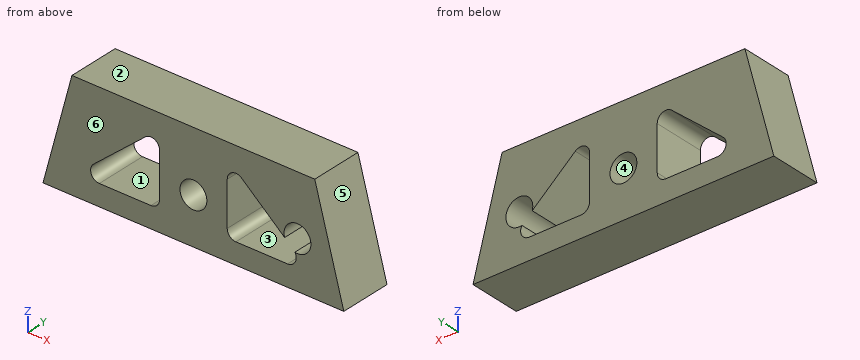
```python
from build123d import *

# Parameters (mm, degrees)
EXTRUDE_1_DEPTH     = 1
EXTRUDE_START       = 5
EXTRUDE_2_DEPTH     = 5
CUT_EXTRUDE_1_REACH = 25.286
SKETCH_2_R          = 1.55
SKETCH_3_R          = 1.55
CUT_EXTRUDE_2_DEPTH = 6


with BuildPart() as part:
    # 草图1 → 凸台-拉伸1 (new body)
    with BuildSketch(Plane(origin=(0, 0, 0), x_dir=(1, 0, 0), z_dir=(0, 1, 0))):
        Polygon((-0.862647581, -12.802774991), (12.834963402, -12.802774991), (16.186049163, -0.402774991), (-18.501877746, -0.402774991), (-15.165036598, -12.802774991), align=None)
        with BuildLine():
            Line((-5.055880083, -8.924536815), (-5.055880083, -3.827423548))
            ThreePointArc((-5.055880083, -3.827423548), (-5.348773301, -3.120316767), (-6.055880083, -2.827423548))
            Line((-6.055880083, -2.827423548), (-12.010923306, -2.827423548))
            ThreePointArc((-12.010923306, -2.827423548), (-12.948929404, -3.480804795), (-12.661184313, -4.587134428))
            Line((-12.661184313, -4.587134428), (-6.70614109, -9.684247695))
            ThreePointArc((-6.70614109, -9.684247695), (-5.63770608, -9.832903758), (-5.055880083, -8.924536815))
        make_face(mode=Mode.SUBTRACT)
        with BuildLine():
            Line((10.34535573, -4.587134428), (4.390312507, -9.684247695))
            ThreePointArc((4.390312507, -9.684247695), (3.321877497, -9.832903758), (2.740051499, -8.924536815))
            Line((2.740051499, -8.924536815), (2.740051499, -3.827423548))
            ThreePointArc((2.740051499, -3.827423548), (3.032944718, -3.120316767), (3.740051499, -2.827423548))
            Line((3.740051499, -2.827423548), (9.695094722, -2.827423548))
            ThreePointArc((9.695094722, -2.827423548), (10.63310082, -3.480804795), (10.34535573, -4.587134428))
        make_face(mode=Mode.SUBTRACT)
    extrude(amount=-EXTRUDE_1_DEPTH)

    # 草图1<8> → 凸台-拉伸2 (add)
    with BuildSketch(Plane(origin=(0, 0, 0), x_dir=(1, 0, 0), z_dir=(0, 1, 0)).offset(EXTRUDE_START)):
        Polygon((-0.862647581, -12.802774991), (12.834963402, -12.802774991), (16.186049163, -0.402774991), (-18.501877746, -0.402774991), (-15.165036598, -12.802774991), align=None)
        with BuildLine():
            Line((-5.055880083, -8.924536815), (-5.055880083, -3.827423548))
            ThreePointArc((-5.055880083, -3.827423548), (-5.348773301, -3.120316767), (-6.055880083, -2.827423548))
            Line((-6.055880083, -2.827423548), (-12.010923306, -2.827423548))
            ThreePointArc((-12.010923306, -2.827423548), (-12.948929404, -3.480804795), (-12.661184313, -4.587134428))
            Line((-12.661184313, -4.587134428), (-6.70614109, -9.684247695))
            ThreePointArc((-6.70614109, -9.684247695), (-5.63770608, -9.832903758), (-5.055880083, -8.924536815))
        make_face(mode=Mode.SUBTRACT)
        with BuildLine():
            Line((10.34535573, -4.587134428), (4.390312507, -9.684247695))
            ThreePointArc((4.390312507, -9.684247695), (3.321877497, -9.832903758), (2.740051499, -8.924536815))
            Line((2.740051499, -8.924536815), (2.740051499, -3.827423548))
            ThreePointArc((2.740051499, -3.827423548), (3.032944718, -3.120316767), (3.740051499, -2.827423548))
            Line((3.740051499, -2.827423548), (9.695094722, -2.827423548))
            ThreePointArc((9.695094722, -2.827423548), (10.63310082, -3.480804795), (10.34535573, -4.587134428))
        make_face(mode=Mode.SUBTRACT)
    extrude(amount=-EXTRUDE_2_DEPTH)

    # 草图2 → 切除-拉伸1 (cut, up to next)
    with BuildSketch(Plane(origin=(0, 5, 0), x_dir=(1, 0, 0), z_dir=(0, 1, 0)), mode=Mode.PRIVATE) as cut_extrude_1_sk1:
        with Locations(Location((-1.157914292, -5.802774991, 0), (0, 0, 270))):
            Circle(SKETCH_2_R)
    cut_extrude_1_tool1 = extrude(cut_extrude_1_sk1.sketch, amount=-CUT_EXTRUDE_1_REACH, mode=Mode.PRIVATE) & part.part
    add(cut_extrude_1_tool1.solids().sort_by_distance((-1.157914, 5, 5.802775))[0], mode=Mode.SUBTRACT)

    # 草图3 → 切除-拉伸2 (cut)
    with BuildSketch(Plane(origin=(0, 5, 0), x_dir=(1, 0, 0), z_dir=(0, 1, 0))):
        with Locations((10.842085708, -5.882306345)):
            Circle(SKETCH_3_R)
    extrude(amount=-CUT_EXTRUDE_2_DEPTH, mode=Mode.SUBTRACT)


solid = part.part
```
Model file for the job. Use its own axes, mm. Face numbers are marked on the shaded views. A direction names the side the tool comes from. Coordinates: 2 decimals unless noted, no trailing zeros. Order: outer loops, then holes, each group sorted by start corner. A loop starts at its lowest first (then second) coordinate and runs counter-clockwise, first axis right, second up. Notation, with made-up numbers: (17.5, 4) -> (42.5, 4) arc R13 ccw to (42.5, 26) -> close; hole circle Ø11 at (70.5, -26). An arc over 180 degrees is marked (long way). Answer as a JSON object with one key per item and string values. Group by question number.
1) Drill centre lines: L1, parallel to X at y = 4.1, z = 5.75; L2, parallel to X at y = 0.25, z = 8; L3, parallel to X at y = 0.7, z = 7. Where is each one in solid material? Low to high.
2) Cut at D-D, the plane x = 12. Write the cut outline in (y, z), then the cut area to 3 significant figures.
3) Cut at A-A, the plane x = -5.5. Write the cut outline in (y, z).
4) Pull direction Z, two halves, no side cores. Call the marked faces 3, 4, 5 and 6: +Z half, -Z half, draft (parallel to the pull), parting line (faces both ways), or undercut.
5) Cut at C-C, the plane z = 8.25. Write the cut outline in (x, y).
6) Flat gauge pins, fed straight in: pin 1 (1 mm diameter, centred on y = 3.5, z = 9.5, fed in from -X); pin 2 (1.5 mm diameter, centred on y = 2, z = 6, fed in from +X); pin 3 (4 mm diameter, centred on x = -1.16, z = 5.8, fed in from -Y); pin 4 (1.5 mm diameter, centred on y = 4, z = 9, fed in from +X). Where does each tip first touch, or does it go through?
7) Cut at B-B, the plane y = 2.75. Write the cut outline in (x, z).
8) Which spindle directions (+Z, -Z, +X, -X, +Y, -Y) get a long thin tool onto all of the face, cutting with end or side? Do the marked faces 1 and 2. Say none if no direction does.
Check values:
{
 "1": {"L1": "x = -17.06 to -11.3, -5.06 to -2.71, 0.39 to 2.74, 8.99 to 9.3, 12.39 to 14.74", "L2": "x = -16.46 to -8.67, -5.06 to 2.74, 6.36 to 14.13", "L3": "x = -16.73 to -9.84, -5.06 to -2.14, -0.17 to 2.74, 7.53 to 9.77, 11.92 to 14.4"},
 "2": {"outline": "(-1, 0.4) -> (5, 0.4) -> (5, 4.85) -> (-1, 4.85) -> close; (-1, 6.91) -> (5, 6.91) -> (5, 12.8) -> (-1, 12.8) -> close", "area": "62.0 mm²"},
 "3": {"outline": "(-1, 0.4) -> (5, 0.4) -> (5, 3) -> (-1, 3) -> close; (-1, 9.76) -> (5, 9.76) -> (5, 12.8) -> (-1, 12.8) -> close"},
 "4": {"face 3": "undercut", "face 4": "undercut", "face 5": "+Z half", "face 6": "draft"},
 "5": {"outline": "(-16.39, -1) -> (-8.38, -1) -> (-8.38, 5) -> (-16.39, 5) -> close; (-5.06, -1) -> (2.74, -1) -> (2.74, 5) -> (-5.06, 5) -> close; (6.07, -1) -> (14.07, -1) -> (14.07, 5) -> (6.07, 5) -> close"},
 "6": {"pin 1": "stops at x = -16.19", "pin 2": "stops at x = 14.88", "pin 3": "stops at y = -1", "pin 4": "stops at x = 14.07"},
 "7": {"outline": "(-18.5, 0.4) -> (16.19, 0.4) -> (12.83, 12.8) -> (-15.17, 12.8) -> close; hole (-12.66, 4.59) arc R1 ccw to (-12.01, 2.83) -> (-6.06, 2.83) arc R1 ccw to (-5.06, 3.83) -> (-5.06, 8.92) arc R1 ccw to (-6.71, 9.68) -> close; hole circle Ø3.1 at (-1.16, 5.8); hole (2.74, 3.83) arc R1 ccw to (3.74, 2.83) -> (9.7, 2.83) arc R1 ccw to (10.54, 4.36) arc R1.55 ccw (long way) to (9.36, 5.43) -> (4.39, 9.68) arc R1 ccw to (2.74, 8.92) -> close"},
 "8": {"face 1": "+Y, -Y", "face 2": "+Z, +X, -X, +Y, -Y"}
}
